Verification items for the finished model (mm, model axes). Face numbers are marked on the shaded views. A direction names the side the tool comes from. Round coordinates to 2 decimals unless told otherwise and drop trailing zeros. Order: outer loops, then holes, each group sorted by start corner. A loop starts at its lowest first (then second) coordinate and runs counter-clockwise, first axis right, second up. Notation, with made-up numbers: (18, 0) -> (65, 0) arc R18 ccw to (65, 16) -> close; hole circle Ø9 at (78.25, 88). An arc over 180 degrees is marked (long way). Put each result on its own line as item: value.
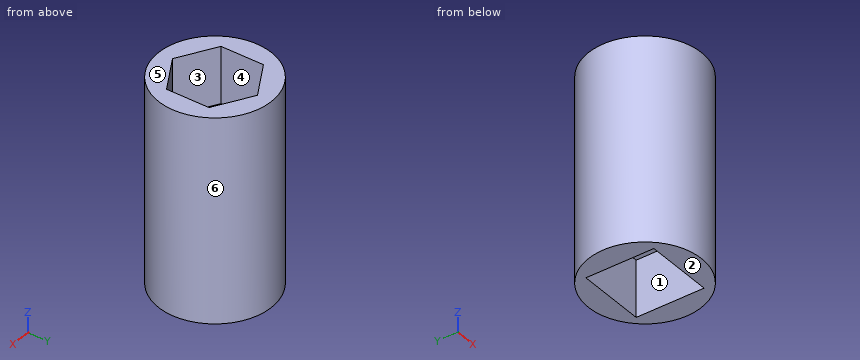
from build123d import *

# Parameters (mm, degrees)
F0_R     = 50
F1_DEPTH = 180
F2_R     = 25
F3_DEPTH = 180
F5_DEPTH = 50
F6_W     = 60
F6_H     = 60
F7_DEPTH = 50


with BuildPart() as f1:
    # F0 (on Top) → F1 (new body)
    with BuildSketch(Plane.XY):
        Circle(F0_R)
    extrude(amount=F1_DEPTH)

    # F2 (on Top) → F3 (cut, through all)
    with BuildSketch(Plane.XY):
        Circle(F2_R)
    extrude(amount=F3_DEPTH, mode=Mode.SUBTRACT)

    # F4 (on face) → F5 (cut)
    with BuildSketch(Plane.XY.offset(180)):
        Polygon((-32.5, 18.763884), (-32.5, -18.763884), (0, -37.527767), (32.5, -18.763884), (32.5, 18.763884), (0, 37.527767), align=None)
    extrude(amount=-F5_DEPTH, mode=Mode.SUBTRACT)

    # F6 (on face) → F7 (cut)
    with BuildSketch(Plane(origin=(0, 0, 0), x_dir=(1, 0, 0), z_dir=(0, 0, -1))):
        Rectangle(F6_W, F6_H)
    extrude(amount=-F7_DEPTH, mode=Mode.SUBTRACT)


solid = f1.part
Item 1: Section check B-B on z = 142. Record the boundary of the cut face in (x, y).
Check sheet entries:
outline: circle Ø100 at (0, 0); hole (-32.5, -18.76) -> (0, -37.53) -> (32.5, -18.76) -> (32.5, 18.76) -> (0, 37.53) -> (-32.5, 18.76) -> close
Item 2: Release check for a two-part mould opening along X. For the marked faces 3, 4, 5 and 6 record: +X half, -X half, draft (parallel to the pull), parting line (faces both ways), or undercut.
Check sheet entries:
face 3: undercut
face 4: undercut
face 5: draft
face 6: parting line
Item 3: Section check D-D on z = 98. Record the boundary of the cut face in (x, y).
Check sheet entries:
outline: circle Ø100 at (0, 0); hole circle Ø50 at (0, 0)
Item 4: Tool access check on the marked faces 1 and 2. Record the directions out of +Z, -Z, +X, -X, +Y, -Y that give a thin tool (end or side, any length) a straight path to the whole face; none if there is none.
Check sheet entries:
face 1: -Z
face 2: -Z, +X, -X, +Y, -Y
Item 5: Section check A-A on y = 0. Record the boundary of the cut face in (x, z), then the cut area to 3 significant figures.
Check sheet entries:
outline: (-50, 0) -> (-30, 0) -> (-30, 50) -> (-25, 50) -> (-25, 130) -> (-32.5, 130) -> (-32.5, 180) -> (-50, 180) -> close; (25, 50) -> (30, 50) -> (30, 0) -> (50, 0) -> (50, 180) -> (32.5, 180) -> (32.5, 130) -> (25, 130) -> close
area: 7,750 mm^2
Item 6: Section check C-C on x = -3. Record the boundary of the cut face in (y, z), then the cut area to 3 significant figures.
Check sheet entries:
outline: (-49.91, 0) -> (-30, 0) -> (-30, 50) -> (-24.82, 50) -> (-24.82, 130) -> (-35.8, 130) -> (-35.8, 180) -> (-49.91, 180) -> close; (24.82, 50) -> (30, 50) -> (30, 0) -> (49.91, 0) -> (49.91, 180) -> (35.8, 180) -> (35.8, 130) -> (24.82, 130) -> close
area: 7,420 mm^2
Item 7: Material ranges on L1, parallel to Y at x = 0, z = 110; L2, parallel to X at y = 14, z = 96; L3, parallel to Y at x = 15, z = 126, recorded low to high. Write a range as [from, to].
Check sheet entries:
L1: y = [-50, -25], [25, 50]
L2: x = [-48, -20.71], [20.71, 48]
L3: y = [-47.7, -20], [20, 47.7]
Item 8: Gauge pin test, flat ends, axial feed: pin 1 Ø6 at (y, z) = (-19.5, 87.5) entering from -X; pin 2 Ø4 at (y, z) = (-6.5, 121) entering from +X; pin 3 Ø2 at (y, z) = (37.5, 148.5) entering from -X. Record the tip position at first contact, or that the pin passes through.
Check sheet entries:
pin 1: stops at x = -47.2
pin 2: stops at x = 49.8
pin 3: stops at x = -34.17
